Geometry check sheet. Reference: the model listing, model coordinates, mm. Face numbers are marked on the shaded views. A direction names the side the tool comes from. Give positions to 0.01 mm unless a question says otherwise; leave off trailing zeros. Write each loop counter-clockwise with the first axis right and the second up, starting at its lowest first coordinate (ties: lowest second). Pieces come first, ordered by that corner, then holes.
(1) Cross-section at A-A (y = -5). Record the boundary of the cut face in (x, z), and give its area (3 significant figures).
(2) Mould release check, pull along X, two halves, no side actions. Record for the marked faces 4 and 5: +X half, -X half, draft (parallel to the pull), parting line (faces both ways), or undercut.
(3) Depth check by flat-ended pin: P1, Ø0.5, axis at y = 24.5, z = 5, coming from the +X side; P2, Ø3.5, axis at x = 7.5, y = -31.5, coming from the +Z side; P3, Ø2.5, axis at y = -39.45, z = 2.72, coming from the -X side; P4, Ø12, axis at y = 12, z = 19, coming from the -X side. Enter the tip coordinate at first touch or a pass-through.
(4) Cross-section at C-C (y = 12). Record the boundary of the cut face in (x, z), and give its area (3 significant figures).
(5) Thickness scan on line 1 along Y through (x, z) = (18, 3.5); line 2 along Y through (x, z) = (-2, 1.25); line 3 along Y through (x, z) = (9.5, 6). Record the ranges inside material, lowest first.
(6) Cross-section at B-B (z = 15). Record the boundary of the cut face in (x, y), and give its area (3 significant figures).
(7) Tool access check on the marked faces 1, 2 and 3. Record the directions out of +Z, -Z, +X, -X, +Y, -Y that give a thin tool (end or side, any length) a straight path to the whole face; none if there is none.
```python
from build123d import *

# Parameters (mm, degrees)
F0_R      = 6.5
F0_W      = 34.999999702
F0_H      = 3
F0_H_2    = 0.3
F1_DEPTH  = 3
F2_DEPTH  = 9.5
F3_DEPTH  = 11.5
F5_DEPTH  = 3
F7_DEPTH  = 3
F8_R      = 1
F9_DEPTH  = 35.000999702
F11_DEPTH = 1
F13_DEPTH = 1
F14_SIZE  = 0.75
F15_W     = 1.8819853365
F15_H     = 1.731043148
F15_W_2   = 1.7636035271
F15_H_2   = 1.938064149
F16_DEPTH = 1
F18_DEPTH = 36.000999702
F19_R     = 1
F20_SIZE2 = 2
F20_SIZE  = 2


# Not quite as in the source:
# - ends of sketch curves that miss each other by under 0.0002 mm in the source are joined
# - a feature names something its author has since deleted; it is built from what else it names


with BuildPart() as f1:
    # F0 (on Top) → F1 (new body)
    with BuildSketch(Plane.XY):
        Polygon((7.8607099131, 16.1003852367), (-9.6392899379, 16.1003852367), (-9.6392899379, -29.3996147633), (25.3607097641, -29.3996147633), (25.3607097641, 16.1003852367), align=None)
        with Locations((7.8607099131, -2.2867515218)):
            Circle(F0_R, mode=Mode.SUBTRACT)
        with Locations((7.8607099131, -31.1996147633)):
            Rectangle(F0_W, F0_H)
        Polygon((-9.6392899379, 19.1003852367), (-9.6392899379, 16.1003852367), (7.8607099131, 16.1003852367), (25.3607097641, 16.1003852367), (25.3607097641, 19.1003852367), (22.192974557, 19.1003852367), (3.3607097641, 19.1003852367), align=None)
        Polygon((-9.6392899379, 46.3003852367), (-9.6392899379, 43.3003852367), (-6.4715547308, 43.3003852367), (12.3607100621, 43.3003852367), (25.3607097641, 43.3003852367), (25.3607097641, 46.3003852367), align=None)
        with Locations((7.8607099131, -29.5496147633)):
            Rectangle(F0_W, F0_H_2)
        Polygon((16.0607097641, 38.1003852367), (25.3607097641, 38.1003852367), (25.3607097641, 43.3003852367), (12.3607100621, 43.3003852367), (12.3607100621, 35.3003852367), (12.3607100621, 34.5003852367), (7.8607097641, 34.5003852367), (7.8607100621, 33.9926332235), (8.7954637781, 33.9926332235), (16.0607097641, 33.9926332235), align=None)
        Polygon((-9.6392899379, 24.3003852367), (-9.6392899379, 19.1003852367), (3.3607097641, 19.1003852367), (3.3607097641, 27.1003852367), (3.3607097641, 27.9003852367), (7.8607100621, 27.9003852367), (7.8607100621, 28.4081372499), (6.9259563461, 28.4081372499), (-0.3392899379, 28.4081372499), (-0.3392899379, 24.3003852367), align=None)
        Polygon((6.9259563461, 34.5003852367), (6.9259563461, 28.4081372499), (7.8607097641, 28.4081372499), (7.8607100621, 33.9926332235), (7.8607100621, 34.5003852367), align=None)
        Polygon((7.8607100621, 28.4081372499), (7.8607100621, 27.9003852367), (8.7954637781, 27.9003852367), (8.7954637781, 33.9926332235), (7.8607097641, 33.9926332235), align=None)
        Polygon((-9.6392899379, 43.3003852367), (-9.6392899379, 24.3003852367), (-0.3392899379, 24.3003852367), (-0.3392899379, 28.4081372499), (6.9259563461, 28.4081372499), (6.9259563461, 34.5003852367), (7.8607100621, 34.5003852367), (12.3607100621, 34.5003852367), (12.3607100621, 35.3003852367), (12.3607100621, 43.3003852367), (-6.4715547308, 43.3003852367), align=None)
        Polygon((3.3607097641, 27.1003852367), (3.3607097641, 19.1003852367), (22.192974557, 19.1003852367), (25.3607097641, 19.1003852367), (25.3607097641, 38.1003852367), (16.0607097641, 38.1003852367), (16.0607097641, 33.9926332235), (8.7954637781, 33.9926332235), (8.7954637781, 27.9003852367), (7.8607100621, 27.9003852367), (3.3607097641, 27.9003852367), align=None)
    extrude(amount=-F1_DEPTH)

    # F0 (on Top) → F2 (join)
    with BuildSketch(Plane.XY):
        with Locations((7.8607099131, -31.1996147633)):
            Rectangle(F0_W, F0_H)
        Polygon((-9.6392899379, 19.1003852367), (-9.6392899379, 16.1003852367), (7.8607099131, 16.1003852367), (25.3607097641, 16.1003852367), (25.3607097641, 19.1003852367), (22.192974557, 19.1003852367), (3.3607097641, 19.1003852367), align=None)
    extrude(amount=F2_DEPTH)

    # F0 (on Top) → F3 (join)
    with BuildSketch(Plane.XY):
        Polygon((-9.6392899379, 46.3003852367), (-9.6392899379, 43.3003852367), (-6.4715547308, 43.3003852367), (12.3607100621, 43.3003852367), (25.3607097641, 43.3003852367), (25.3607097641, 46.3003852367), align=None)
        Polygon((-9.6392899379, 24.3003852367), (-9.6392899379, 19.1003852367), (3.3607097641, 19.1003852367), (3.3607097641, 27.1003852367), (3.3607097641, 27.9003852367), (7.8607100621, 27.9003852367), (7.8607100621, 28.4081372499), (6.9259563461, 28.4081372499), (-0.3392899379, 28.4081372499), (-0.3392899379, 24.3003852367), align=None)
        Polygon((7.8607100621, 28.4081372499), (7.8607100621, 27.9003852367), (8.7954637781, 27.9003852367), (8.7954637781, 33.9926332235), (7.8607097641, 33.9926332235), align=None)
        Polygon((6.9259563461, 34.5003852367), (6.9259563461, 28.4081372499), (7.8607097641, 28.4081372499), (7.8607100621, 33.9926332235), (7.8607100621, 34.5003852367), align=None)
        Polygon((16.0607097641, 38.1003852367), (25.3607097641, 38.1003852367), (25.3607097641, 43.3003852367), (12.3607100621, 43.3003852367), (12.3607100621, 35.3003852367), (12.3607100621, 34.5003852367), (7.8607097641, 34.5003852367), (7.8607100621, 33.9926332235), (8.7954637781, 33.9926332235), (16.0607097641, 33.9926332235), align=None)
        Polygon((-9.6392899379, 19.1003852367), (-9.6392899379, 16.1003852367), (7.8607099131, 16.1003852367), (25.3607097641, 16.1003852367), (25.3607097641, 19.1003852367), (22.192974557, 19.1003852367), (3.3607097641, 19.1003852367), align=None)
    extrude(amount=F3_DEPTH)

    # F4 (on face) → F5 (join)
    with BuildSketch(Plane.YZ.offset(25.3607097641)):
        Polygon((-32.6996147633, -3), (46.3003852367, -3), (46.3003852367, 11.5), (38.1003852367, 11.5), (38.1003852367, 0), (19.1003852367, 0), (19.1003852367, 11.5), (16.1003852367, 11.5), (16.1003852367, 0), (-29.6996147633, 0), (-29.6996147633, 9.5), (-32.6996147633, 9.5), align=None)
        with BuildLine():
            Line((46.3003852367, 11.5), (46.3003852367, -3))
            Line((46.3003852367, -3), (60.2135883006, 16.6053474951))
            ThreePointArc((60.2135883006, 16.6053474951), (54.0324103863, 15.4756413664), (52.7478740756, 21.6265082006))
            Line((52.7478740756, 21.6265082006), (46.3003852367, 11.5))
        make_face()
        with BuildLine():
            ThreePointArc((52.7478740756, 21.6265082006), (54.0324103863, 15.4756413664), (60.2135883006, 16.6053474951))
            ThreePointArc((60.2135883006, 16.6053474951), (60.8312132136, 17.8429507129), (61.0437823534, 19.2096754909))
            ThreePointArc((61.0437823534, 19.2096754909), (57.8024349564, 23.5300682537), (52.7478740756, 21.6265082006))
        make_face()
        with BuildLine():
            Line((-40.2101505455, -1.7121333681), (-32.6996147633, -3))
            Line((-32.6996147633, -3), (-32.6996147633, 9.5))
            Line((-32.6996147633, 9.5), (-40.7689799002, 7.0253734949))
            ThreePointArc((-40.7689799002, 7.0253734949), (-36.7744645914, 6.3416367755), (-34.9496147633, 2.7231327258))
            ThreePointArc((-34.9496147633, 2.7231327258), (-36.5489606146, -0.7172459612), (-40.2101505455, -1.7121333681))
        make_face()
        with BuildLine():
            ThreePointArc((-40.7689799002, 7.0253734949), (-43.9404391312, 2.4359106929), (-40.2101505455, -1.7121333681))
            ThreePointArc((-40.2101505455, -1.7121333681), (-36.5489606146, -0.7172459612), (-34.9496147633, 2.7231327258))
            ThreePointArc((-34.9496147633, 2.7231327258), (-36.7744645914, 6.3416367755), (-40.7689799002, 7.0253734949))
        make_face()
    extrude(amount=-F5_DEPTH)

    # F6 (on face) → F7 (join)
    with BuildSketch(Plane(origin=(-9.6392899379, 0, 0), x_dir=(0, -1, 0), z_dir=(-1, 0, 0))):
        with BuildLine():
            Line((-60.2135883006, 16.6053474951), (-46.3003852367, -3))
            Line((-46.3003852367, -3), (-46.3003852367, 11.5))
            Line((-46.3003852367, 11.5), (-52.7478740756, 21.6265082006))
            ThreePointArc((-52.7478740756, 21.6265082006), (-59.0551543205, 22.9437096154), (-60.2135883006, 16.6053474951))
        make_face()
        Polygon((-46.3003852367, 11.5), (-46.3003852367, -3), (32.6996147633, -3), (32.6996147633, 9.5), (29.6996147633, 9.5), (29.6996147633, 0), (-16.1003852367, 0), (-16.1003852367, 11.5), (-24.3003852367, 11.5), (-24.3003852367, 0), (-43.3003852367, 0), (-43.3003852367, 11.5), align=None)
        with BuildLine():
            Line((32.6996147633, 9.5), (32.6996147633, -3))
            Line((32.6996147633, -3), (40.2101505455, -1.7121333681))
            ThreePointArc((40.2101505455, -1.7121333681), (43.9404391312, 2.4359106929), (40.7689799002, 7.0253734949))
            Line((40.7689799002, 7.0253734949), (32.6996147633, 9.5))
        make_face()
    extrude(amount=-F7_DEPTH)

    # F8 (on face) → F9 (cut, through all)
    with BuildSketch(Plane(origin=(-9.6392899379, 0, 0), x_dir=(0, -1, 0), z_dir=(-1, 0, 0))):
        with Locations((-56.5437823534, 19.2096754909)):
            Circle(F8_R)
        with Locations((39.4496147633, 2.7231327258)):
            Circle(F8_R)
    extrude(amount=-F9_DEPTH, mode=Mode.SUBTRACT)

    # F10 (on face) → F11 (join)
    with BuildSketch(Plane.YZ.offset(25.3607097641)):
        Polygon((39.4906885922, 7.75), (38.1003852367, 7.75), (38.1003852367, 3.75), (39.4906885922, 3.75), (39.4906885922, 5.75), align=None)
        Polygon((38.1003852367, 3.75), (38.1003852367, 7.75), (37.4906885922, 7.75), (37.4906885922, 5.75), (37.4906885922, 3.75), align=None)
    extrude(amount=F11_DEPTH)

    # F12 (on face) → F13 (join)
    with BuildSketch(Plane(origin=(-9.6392899379, 0, 0), x_dir=(0, -1, 0), z_dir=(-1, 0, 0))):
        Polygon((-22.9083076119, 7.75), (-24.3003852367, 7.75), (-24.3003852367, 3.75), (-22.9083076119, 3.75), (-22.9083076119, 5.75), align=None)
        Polygon((-24.9083076119, 7.75), (-24.9083076119, 5.75), (-24.9083076119, 3.75), (-24.3003852367, 3.75), (-24.3003852367, 7.75), align=None)
    extrude(amount=F13_DEPTH)

    # F14
    f14_edges = [f1.edges().sort_by_distance(p)[0] for p in [
        (-10.63929, 24.908308, 5.75),
        (-10.63929, 22.908308, 5.75),
        (-10.63929, 23.908308, 7.75),
        (-10.63929, 23.908308, 3.75),
        (26.36071, 38.490689, 7.75),
        (26.36071, 37.490689, 5.75),
        (26.36071, 38.490689, 3.75),
        (26.36071, 39.490689, 5.75),
    ]]
    chamfer(f14_edges, length=F14_SIZE)

    # F15 (on face) → F16 (join)
    with BuildSketch(Plane.XY.offset(11.5)):
        with Locations((11.4197173938, 35.3659068108)):
            Rectangle(F15_W, F15_H)
        with Locations((4.2425115276, 26.9313531622)):
            Rectangle(F15_W_2, F15_H_2)
    extrude(amount=-F16_DEPTH)

    # F17 (on face) → F18 (cut, through all)
    with BuildSketch(Plane(origin=(-9.6392899379, 0, 0), x_dir=(0, -1, 0), z_dir=(-1, 0, 0))):
        with BuildLine():
            Line((-56.1974216606, 10.9460940352), (-46.3003852367, -3))
            Line((-46.3003852367, -3), (-32.2360508144, -3))
            add(Edge.make_bspline(
                [(-56.1974216606, 10.9460940352), (-49.7821666885, 1.9062415714), (-46.3003852367, -3), (-32.2360508144, -3)],
                knots=[0, 0, 0, 0, 27.7243725207, 27.7243725207, 27.7243725207, 27.7243725207], degree=3))
        make_face()
    extrude(amount=-F18_DEPTH, mode=Mode.SUBTRACT)

    # F19
    f19_edges = [f1.edges().sort_by_distance(p)[0] for p in [
        (5.124313, 25.962321, 11),
        (10.478725, 36.231428, 11),
    ]]
    fillet(f19_edges, radius=F19_R)

    # F20
    f20_edges = [f1.edges().sort_by_distance(p)[0] for p in [
        (7.86071, 16.100385, 11.5),
    ]]
    chamfer(f20_edges, length=F20_SIZE, length2=F20_SIZE2)


solid = f1.part
```
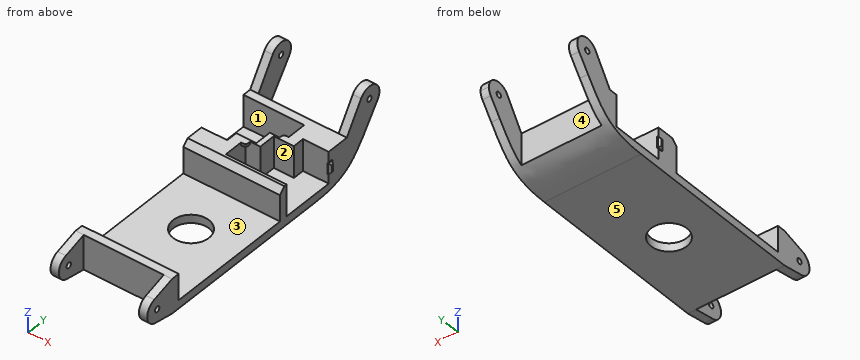
Reply:
1. outline: (-9.64, -3) - (1.95, -3) - (1.95, 0) - (-9.64, 0) - close; (13.77, -3) - (25.36, -3) - (25.36, 0) - (13.77, 0) - close
1. area: 69.6 mm2
2. face 4: undercut
2. face 5: draft
3. P1: stops at x = 3.36
3. P2: stops at z = 9.5
3. P3: stops at x = -9.64
3. P4: passes through
4. outline: (-9.64, -3) - (25.36, -3) - (25.36, 0) - (-9.64, 0) - close
4. area: 105 mm2
5. line 1: y = -32.7 to -29.7, 16.1 to 19.1, 38.1 to 46.3
5. line 2: y = -32.7 to -29.7, 16.1 to 24.3, 43.3 to 46.3
5. line 3: y = -32.7 to -29.7, 16.1 to 19.1, 33.99 to 34.5, 43.3 to 46.3
6. outline: (-9.64, 48.53) - (-6.64, 48.53) - (-6.64, 59.07) - (-9.64, 59.07) - close; (22.36, 48.53) - (25.36, 48.53) - (25.36, 59.07) - (22.36, 59.07) - close
6. area: 63.3 mm2
7. face 1: +Z, -X
7. face 2: +Z, +X
7. face 3: +Z, +X, -X
